CAD build for the part. Positions are in the model's coordinates, mm. A direction names the side the tool comes from. Give positions to 0.01 mm unless a question says otherwise; leave off trailing zeros. Loops run counter-clockwise (first coordinate to the right, second up) from the corner with the lowest first, then second, coordinate; pieces in that order, holes last. Notation, with made-up numbers: M -30.75,29.25 L 19.25,29.25 A15 cw 19.25,33.25 Z; hole C -38,-13 d4. An arc over 180 degrees is marked long. Answer as CSV lines item,"result".
Autodesk Inventor part; units mm, degrees
ref_plane "YZ Plane" through (0, 0, 0) normal (1, 0, 0) x (0, 1, 0)
ref_plane "XZ Plane" through (0, 0, 0) normal (0, 1, 0) x (-1, 0, 0)
ref_plane "XY Plane" through (0, 0, 0) normal (0, 0, 1) x (1, 0, 0)
sketch "草圖1" plane through (0, 0, 0) normal (0, 1, 0) x (-1, 0, 0)
  line L0 (0, 0) -> (-24, 0)
  line L1 (-24, 0) -> (-24, -14)
  line L2 (-24, -14) -> (-48, -14)
  line L3 (-48, -14) -> (-48, -38)
  line L4 (-48, -38) -> (0, -38)
  line L5 (0, -38) -> (0, 0)
  dimension "d0" = 24
  dimension "d1" = 14
  dimension "d2" = 38
  dimension "d3" = 48
extrude "擠出1" add sketch "草圖1" along normal blind 12
sketch "草圖2" plane through (48, 0, -38) normal (0, 0, -1) x (-1, 0, 0)
  line L0 (48, 12) -> (24, 12)
  line L1 (48, 12) -> (48, 24)
  line L2 (48, 24) -> (24, 24)
  line L3 (24, 24) -> (24, 36)
  line L4 (24, 36) -> (12, 36)
  line L5 (12, 36) -> (0, 24)
  line L6 (24, 12) -> (0, 12)
  line L7 (0, 24) -> (0, 12)
  line L8 (0, 12) -> (48, 12)
  point P0 (48, 0)
  dimension "d6" = 12
  dimension "d7" = 24
  dimension "d8" = 12
  dimension "d9" = 12
extrude "擠出2" add sketch "草圖2" against normal blind 14
properties part number "410571040練習一"
1) Flat gauge pins, fed straight in: pin 1 (4 mm diameter, centred on x = 36.5, z = -30.5, fed in from -Y); pin 2 (9.5 mm diameter, centred on x = 32, y = 9, fed in from +Z); pin 3 (11 mm diameter, centred on x = 12.5, z = -31.5, fed in from +Y); pin 4 (7 mm diameter, centred on x = 17.5, z = -13.5, fed in from +Y). Where does each tip first touch, or does it go through?
Answer below:
pin 1,"stops at y = 0"
pin 2,"stops at z = -14"
pin 3,"stops at y = 24"
pin 4,"stops at y = 12"
2) Band-saw the part on D-D on y = 33.5. Give the cut face in (x, z).
Answer below:
outline,"M 24,-38 L 38.5,-38 L 38.5,-24 L 24,-24 Z"
3) Band-saw the part on A-A on z = -25. Give the cut face in (x, y).
Answer below:
outline,"M 0,0 L 48,0 L 48,24 L 36,36 L 24,36 L 24,24 L 0,24 Z"
4) Which spindle directions (+Z, -Z, +X, -X, +Y, -Y) get a long thin tool onto all of the face, cutting with end or side? Do faces 1 (the face through (30, 22, -24)), 2 (the face through (24, 30, -31)), 3 (the face through (24, 6, -7)), 4 (the face through (12, 6, 0)), 5 (the face through (24, 0, -23)). Say none if no direction does.
Answer below:
face 1,"+Z, +X, -X, +Y"
face 2,"+Z, -Z, -X, +Y"
face 3,"+Z, +X, +Y, -Y"
face 4,"+Z, +X, -X, +Y, -Y"
face 5,"+Z, -Z, +X, -X, -Y"
5) Mould opens along X. For faces 6 (the face through (0, 9, -23)), 7 (the face through (12, 24, -31)), 8 (the face through (42, 30, -31)) say: +X half, -X half, draft (parallel to the pull), parting line (faces both ways), or undercut.
Answer below:
face 6,"-X half"
face 7,"draft"
face 8,"+X half"
6) Drill centre lines: line 1 (Y direction, x = 23, z = -22); line 2 (Z direction, x = 17.5, y = 12.5); line 3 (Z direction, x = 27.5, y = 2). Where is each one in solid material? Low to high. Write a range as from..to.
Answer below:
line 1,"y = 0..12"
line 2,"z = -38..-24"
line 3,"z = -38..-14"
7) Band-saw the part on B-B on y = 8. Give the cut face in (x, z).
Answer below:
outline,"M 0,-38 L 48,-38 L 48,-14 L 24,-14 L 24,0 L 0,0 Z"
8) Band-saw the part on C-C on x = 26. Give the cut face in (y, z), and give its area (3 significant figures).
Answer below:
outline,"M 0,-38 L 36,-38 L 36,-24 L 12,-24 L 12,-14 L 0,-14 Z"
area,"624 mm^2"
